Source: CAD feature listing. Evaluate the final solid. Frame: model axes, mm. A direction names the side the tool comes from. Give positions to 0.01 mm unless a question says otherwise; leave off trailing zeros. Loops run counter-clockwise (first coordinate to the right, second up) from the corner with the lowest first, then second, coordinate; pieces in that order, holes last. Notation, with made-up numbers: (89.25, -27) -> (99.25, -27) arc R16 ccw to (99.25, -20) -> close; hole circle Ø8 at (62, 58). An arc over 180 degrees is marked (long way). Put each result on its own line as item: value.
```python
from build123d import *

# Parameters (mm, degrees)
BOSS_EXTRUDE1_START = 1
SKETCH1_R           = 5
BOSS_EXTRUDE1_DEPTH = 14
CUT_EXTRUDE1_START  = -1.5
SKETCH2_W           = 2.15
SKETCH2_H           = 6.2
CUT_EXTRUDE1_DEPTH  = 15
FILLET2_R           = 1
SKETCH3_W           = 10
SKETCH3_H           = 1
CUT_EXTRUDE2_DEPTH  = 0.5


with BuildPart() as part:
    # Sketch1 → Boss-Extrude1 (new body)
    with BuildSketch(Plane.XY.offset(BOSS_EXTRUDE1_START)):
        with Locations((15.441970815, -61.974353767)):
            Circle(SKETCH1_R)
    extrude(amount=BOSS_EXTRUDE1_DEPTH)

    # Sketch2 → Cut-Extrude1 (cut)
    with BuildSketch(Plane.XY.offset(15).offset(CUT_EXTRUDE1_START)):
        with Locations((15.441970815, -61.974353767)):
            Rectangle(SKETCH2_W, SKETCH2_H)
    extrude(amount=-CUT_EXTRUDE1_DEPTH, mode=Mode.SUBTRACT)

    # Fillet2
    fillet2_edges = [part.edges().sort_by_distance(p)[0] for p in [
        (10.441970815, -61.974353767, 15),
    ]]
    fillet(fillet2_edges, radius=FILLET2_R)

    # Sketch3 → Cut-Extrude2 (cut)
    with BuildSketch(Plane.XY.offset(15)):
        with Locations((15.441970815, -61.974353767)):
            Rectangle(SKETCH3_W, SKETCH3_H)
    extrude(amount=-CUT_EXTRUDE2_DEPTH, mode=Mode.SUBTRACT)


solid = part.part
```
(1) Draft query along X for faces 1 (the flat face through (15, -65.074, 7)), 2 (the cylindrical face through (20.06, -63.89, 7.41)), 3 (the flat face through (15, -62, 14.5)). Return one class per face: released by +X, released by -X, zero draft, split by the parting line, or undercut.
Calculated:
face 1: undercut
face 2: split by the parting line
face 3: zero draft
(2) Line query: probe 1 along Y at (x, z) = (15.5, 12); probe 2 along X at (y, z) = (-61, 11.5); probe 3 along X at (y, z) = (-60, 10). Output: solid intervals per line, ascending. Write a range as from..to.
Calculated:
probe 1: y = -66.97..-65.07, -58.87..-56.97
probe 2: x = 10.54..14.37, 16.52..20.35
probe 3: x = 10.85..14.37, 16.52..20.04
(3) Reachability of faces 4 (the flat face through (15, -64, 15)), 5 (the flat face through (15, -58.874, 7)) from +Z, -Z, +X, -X, +Y, -Y: full face, straight path, thin tool, end or side. Return the list, or none.
Calculated:
face 4: +Z, +X, -X, +Y, -Y
face 5: -Z
(4) First-contact query: P1, Ø5, axis at y = -59.5, z = 12.5, coming from the +X side; P2, Ø1.5, axis at x = 16.5, z = 8.5, coming from the +Y side; P3, Ø0.5, axis at x = 16, y = -62, coming from the +Z side. Flat tips, straight axial feed; report the tip coordinate or a pass-through.
Calculated:
P1: stops at x = 20.44
P2: stops at y = -56.98
P3: stops at z = 14.5
(5) Section A-A on z = 6.75. Return loops of the section in (x, y).
Calculated:
outline: circle Ø10 at (15.44, -61.97); hole (14.37, -65.07) -> (16.52, -65.07) -> (16.52, -58.87) -> (14.37, -58.87) -> close
